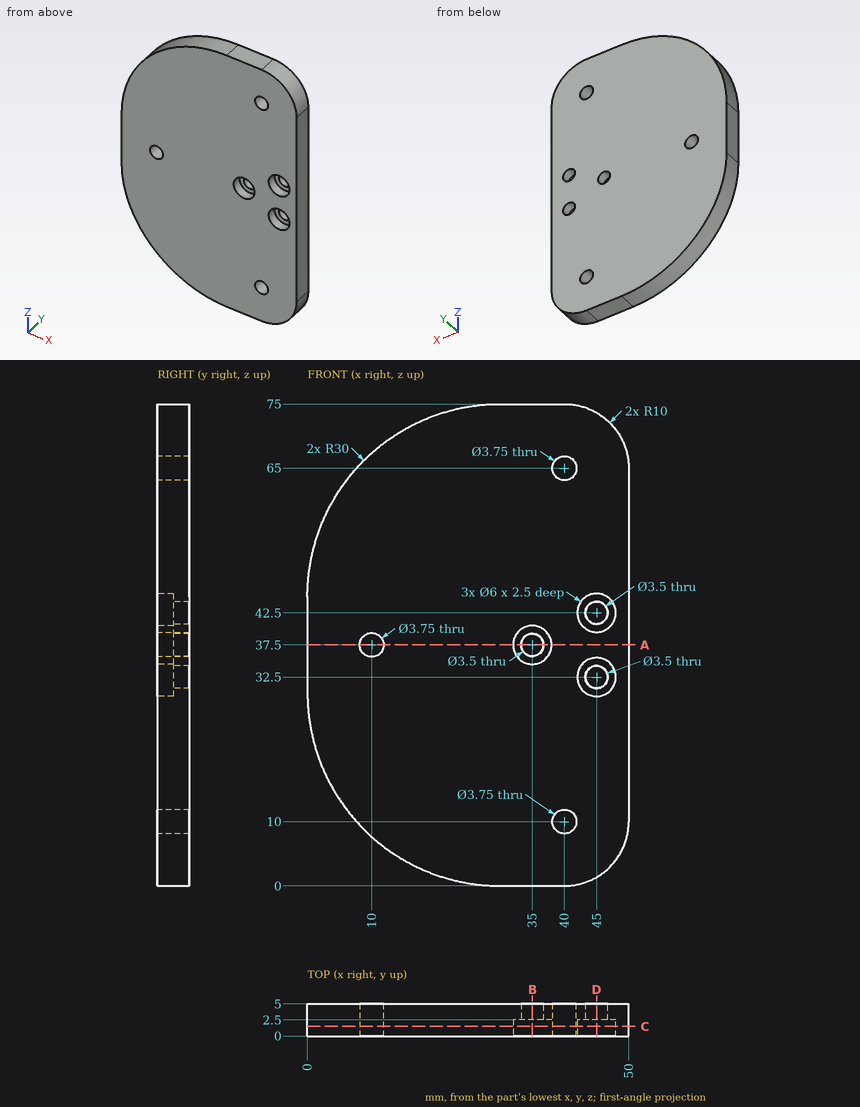
Here's the drawing with two shaded views (mm, measured from the low corner). I have some questions. Round coordinates to 2 decimals unless told otherwise and drop trailing zeros. Write each loop counter-clockwise with the first axis right and the second up, starting at its lowest first coordinate (ties: lowest second). Pieces come first, ordered by that corner, then holes. Notation, with made-up numbers: M 58,49 L 79,49 A20 cw 79,60 Z; hole C 40.5,88.25 d5. An arc over 180 degrees is marked long. Answer in a Markdown table with one row per item. Add a question column.
Q1. If I drill on line 1 (Z direction, x = 45, y = 1.1); line 2 (Z direction, x = 45, y = 3.2); line 3 (X direction, y = 3.7, z = 42.5), over which ranges is the centre line in solid material (lowest first)? Write a range as from..to.
Q2. Imagine slicing it at B-B (x = 35). Please give me the cut outline in (y, z).
Q3. Imagine slicing it at C-C (y = 1.5). Please give me the cut outline in (x, z) (3 decimals).
Q4. Will these pins go through, and if not, where does the flat tip stop? pin 1 Ø3 at (x, z) = (45, 42.5) entering from -Y; pin 2 Ø1.8 at (x, z) = (33.5, 37) entering from -Y.
Q5. Imagine slicing it at A-A (z = 37.5). Please give me the cut outline in (x, y) (3 decimals).
Q6. Imagine slicing it at D-D (x = 45). Please give me the cut outline in (y, z), then the cut area to 3 significant figures.
Values:
| question | item | result |
|---|---|---|
| 1 | line 1 | 1.34..29.5, 35.5..39.5, 45.5..73.66 |
| 1 | line 2 | 1.34..30.75, 34.25..40.75, 44.25..73.66 |
| 1 | line 3 | 0..43.25, 46.75..50 |
| 2 | outline | M 0,0 L 5,0 L 5,35.75 L 2.5,35.75 L 2.5,34.5 L 0,34.5 Z; M 0,40.5 L 2.5,40.5 L 2.5,39.25 L 5,39.25 L 5,75 L 0,75 Z |
| 3 | outline | M 0,30 A30 ccw 30,0 L 40,0 A10 ccw 50,10 L 50,65 A10 ccw 40,75 L 30,75 A30 ccw 0,45 Z; hole C 10,37.5 d3.75; hole C 35,37.5 d6; hole C 40,10 d3.75; hole C 40,65 d3.75; hole C 45,32.5 d6; hole C 45,42.5 d6 |
| 4 | pin 1 | through |
| 4 | pin 2 | y = 2.5 |
| 5 | outline | M 0,0 L 8.125,0 L 8.125,5 L 0,5 Z; M 11.875,0 L 32,0 L 32,2.5 L 33.25,2.5 L 33.25,5 L 11.875,5 Z; M 36.75,2.5 L 38,2.5 L 38,0 L 50,0 L 50,5 L 36.75,5 Z |
| 6 | outline | M 0,1.34 L 5,1.34 L 5,30.75 L 2.5,30.75 L 2.5,29.5 L 0,29.5 Z; M 0,35.5 L 2.5,35.5 L 2.5,34.25 L 5,34.25 L 5,40.75 L 2.5,40.75 L 2.5,39.5 L 0,39.5 Z; M 0,45.5 L 2.5,45.5 L 2.5,44.25 L 5,44.25 L 5,73.66 L 0,73.66 Z |
| 6 | area | 314 mm^2 |
